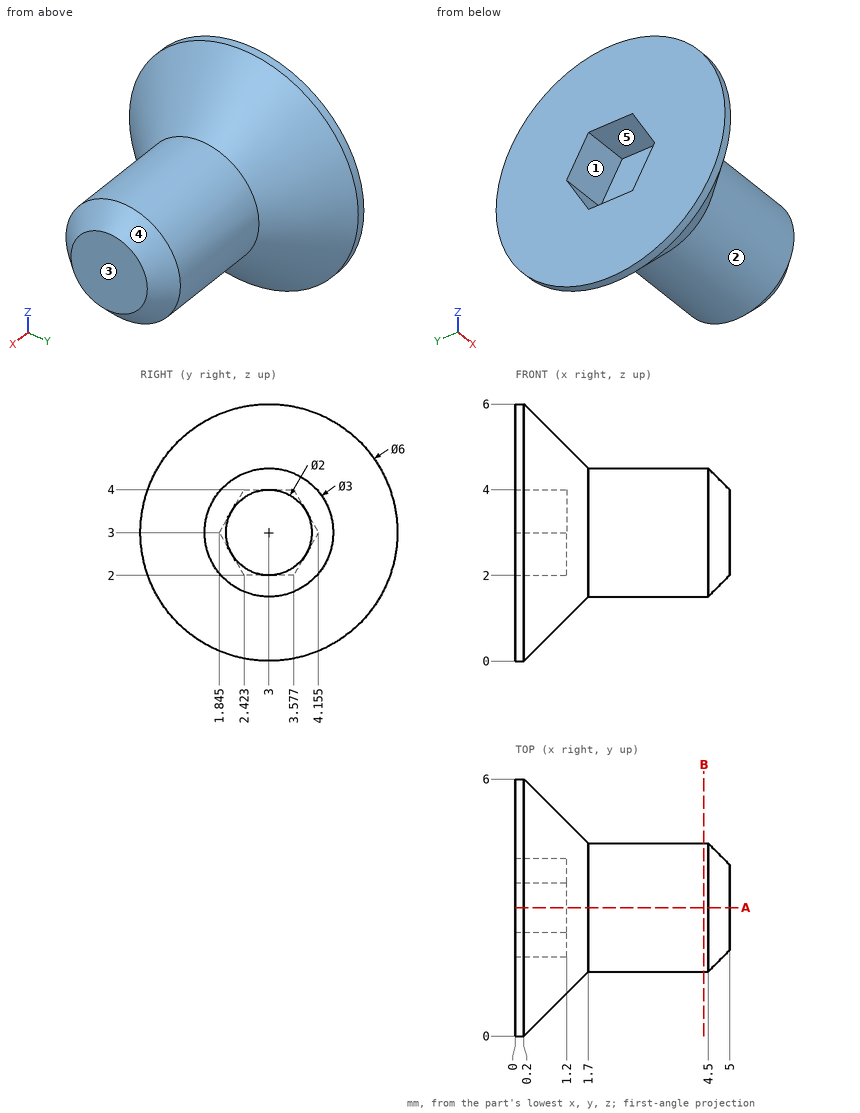
Input: dimensioned drawing with shaded views. Units: mm. Origin: part minimum x, y, z. A direction names the side the tool comes from. Coordinates: 2 decimals unless noted, no trailing zeros. Write each loop counter-clockwise with the first axis right and the second up, starting at its lowest first coordinate (ties: lowest second). Pieces come first, ordered by that corner, then holes. Notation, with made-up numbers: M -1,62 L 5,62 A28 cw 5,98 Z; hole C 3.5,39 d10. An arc over 180 degrees is marked long. Answer as CSV lines item,"result". Start each with the question number.
Q1. Reachability of the marked faces 4 and 5 from +Z, -Z, +X, -X, +Y, -Y: full face, straight path, thin tool, end or side. Return the list, or none.
Q2. Mould query, pull axis Y, two halves, no side actions, for the marked faces 1, 2 and 3. Classes: released by +Y, released by -Y, zero draft, split by the parting line, or undercut.
Q3. Line query: line 1 (Z direction, x = 0.3, y = 4) (1 decimal); line 2 (Y direction, x = 0.55, z = 2.8); line 3 (Y direction, x = 1.25, z = 3.8). Output: solid intervals per line, ascending. Write a range as from..to.
Q4. Cut plane B-B on x = 4.4. Return the cut outline in (y, z).
Q5. Cut plane A-A on y = 3. Return the cut outline in (x, z).
Q6. Pin query (flat end, axial travel): P1, Ø1, axis at x = 1, y = 4.5, coming from the +Z side; P2, Ø1.5, axis at x = 1, y = 3, coming from the -Z side; P3, Ø2, axis at x = 4, z = 2.5, coming from the +Y side. Return the tip coordinate at first contact, or that it passes through.
Findings below:
1,face 4,"+X"
1,face 5,"-X"
2,face 1,"undercut"
2,face 2,"split by the parting line"
2,face 3,"zero draft"
3,line 1,"z = 0.3..2.7, 3.3..5.7"
3,line 2,"y = 0.36..1.96, 4.04..5.64"
3,line 3,"y = 1.22..4.78"
4,outline,"C 3,3 d3"
5,outline,"M 0,0 L 0.2,0 L 1.7,1.5 L 4.5,1.5 L 5,2 L 5,4 L 4.5,4.5 L 1.7,4.5 L 0.2,6 L 0,6 L 0,4 L 1.2,4 L 1.2,2 L 0,2 Z"
6,P1,"stops at z = 5.32"
6,P2,"stops at z = 0.05"
6,P3,"stops at y = 4.5"
